```python
from build123d import *

# Parameters (mm, degrees)
SKETCH1_W           = 30
SKETCH1_H           = 28
BOSS_EXTRUDE1_DEPTH = 15
CUT_EXTRUDE4_DEPTH  = 44.69210455
SKETCH3_W           = 5
SKETCH3_H           = 15
EXTRUDE_3_DEPTH     = 30


with BuildPart() as part:
    # Sketch1 → Boss-Extrude1 (new body)
    with BuildSketch(Plane.XY):
        with Locations((15, -14)):
            Rectangle(SKETCH1_W, SKETCH1_H)
    extrude(amount=-BOSS_EXTRUDE1_DEPTH)

    # Sketch2 → Cut-Extrude4 (cut, through all)
    with BuildSketch(Plane.XY):
        Polygon((23, 0), (15, -6), (7, 0), align=None)
    extrude(amount=-CUT_EXTRUDE4_DEPTH, mode=Mode.SUBTRACT)

    # Sketch3 → 凸台-拉伸3 (add)
    with BuildSketch(Plane.XY):
        with Locations((-2.5, -20.5)):
            Rectangle(SKETCH3_W, SKETCH3_H)
        with Locations((2.5, -20.5)):
            Rectangle(SKETCH3_W, SKETCH3_H)
        with Locations((27.5, -20.5)):
            Rectangle(SKETCH3_W, SKETCH3_H)
        with Locations((32.5, -20.5)):
            Rectangle(SKETCH3_W, SKETCH3_H)
    extrude(amount=-EXTRUDE_3_DEPTH)


solid = part.part
```
Input: part model. Units: mm. Frame: model coordinates. A direction names the side the tool comes from. Give positions to 0.01 mm unless a question says otherwise; leave off trailing zeros. Loops run counter-clockwise (first coordinate to the right, second up) from the corner with the lowest first, then second, coordinate; pieces in that order, holes last.
1) Section query A-A on z = -26. Return the cut outline in (x, y).
A:
outline: (-5, -28) - (5, -28) - (5, -13) - (-5, -13) - close; (25, -28) - (35, -28) - (35, -13) - (25, -13) - close
2) Line query: L1, parallel to X at y = -26, z = -19.5; L2, parallel to Y at x = 2, z = -22.25; L3, parallel to Z at x = 7, y = -26.5. Output: solid intervals per line, ascending.
A:
L1: x = -5 to 5, 25 to 35
L2: y = -28 to -13
L3: z = -15 to 0
3) Section query C-C on z = -4. Return the cut outline in (x, y), and give its area (3 significant figures).
A:
outline: (-5, -28) - (35, -28) - (35, -13) - (30, -13) - (30, 0) - (23, 0) - (15, -6) - (7, 0) - (0, 0) - (0, -13) - (-5, -13) - close
area: 942 mm2
4) Section query B-B on y = -3.25. Return the cut outline in (x, z).
A:
outline: (0, -15) - (11.33, -15) - (11.33, 0) - (0, 0) - close; (18.67, -15) - (30, -15) - (30, 0) - (18.67, 0) - close
5) Reachability of faces 1 (the flat face through (25, -21, -22)), 2 (the flat face through (19, -3, -7)), 3 (the flat face through (35, -21, -15)), 4 (the flat face through (0, -7, -7)), 5 (the flat face through (30, -7, -7)) from +Z, -Z, +X, -X, +Y, -Y: full face, straight path, thin tool, end or side. Return the list, or none.
A:
face 1: -Z, +Y, -Y
face 2: +Z, -Z, +Y
face 3: +Z, -Z, +X, +Y, -Y
face 4: +Z, -Z, -X, +Y
face 5: +Z, -Z, +X, +Y
6) Contact query for flat-ended pins moving along their axis: pin 1 (3 mm diameter, centred on x = 29.5, z = -21, fed in from +Y); pin 2 (6.5 mm diameter, centred on y = -9, z = -10.5, fed in from +X); pin 3 (6.5 mm diameter, centred on y = -5, z = -7.5, fed in from -X). Output: stop coordinate, or through.
A:
pin 1: stops at y = -13
pin 2: stops at x = 30
pin 3: stops at x = 0
7) Section query D-D on y = -20.5. Return the cut outline in (x, z).
A:
outline: (-5, -30) - (5, -30) - (5, -15) - (25, -15) - (25, -30) - (35, -30) - (35, 0) - (-5, 0) - close
8) Mould query, pull axis X, two halves, no side actions, for faces 6 (the flat face through (-5, -21, -15)), 7 (the flat face through (15, -28, -11)), 8 (the flat face through (11, -3, -7)). Classes: released by +X, released by -X, zero draft, split by the parting line, or undercut.
A:
face 6: released by -X
face 7: zero draft
face 8: undercut
